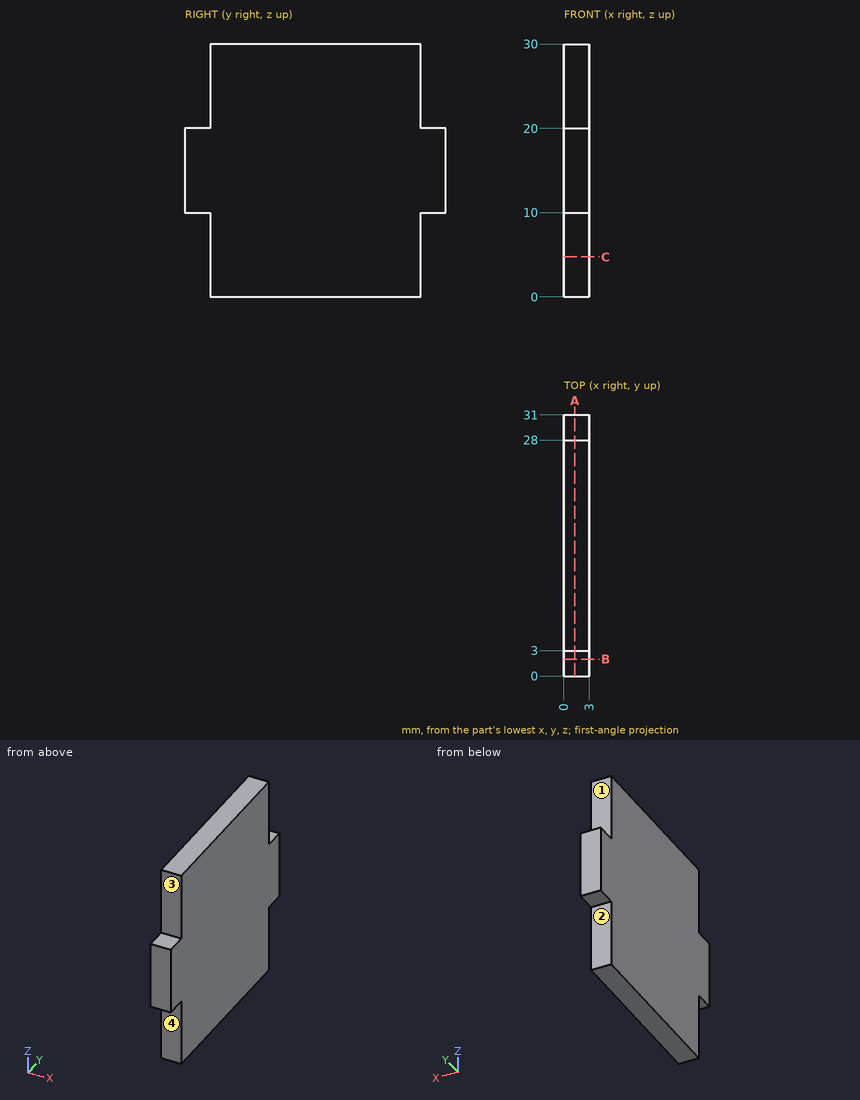
The figure shows three views and two pictorial views of one solid part (mm, origin at its lowest corner). Answer the questions. A direction names the side the tool comes from. Give positions to 0.01 mm unless a question says otherwise; leave off trailing zeros. Write each loop counter-clockwise with the first axis right and the second up, starting at its lowest first coordinate (ties: lowest second). Pieces come first, ordered by that corner, then holes. Notation, with made-up numbers: (-16.5, 63) - (-6.5, 63) arc R21 ccw to (-6.5, 78) - close; hole circle Ø11 at (33.25, 71.5). An arc over 180 degrees is marked (long way). Use one line per item in the form item = value. Start each with the question number.
1) A tool of negligible diameter and unlimited length cuts with its end or side. For the marked faces 1, 2, 3 and 4, from which of +Z, -Z, +X, -X, +Y, -Y can it reach the whole face along a straight path? Write none if from no direction.
2) Find section C-C on z = 4.75. Determine the outline of the cut face in (x, y), plus the area to 3 significant figures.
3) Find section B-B on y = 2. Determine the outline of the cut face in (x, z), plus the area to 3 significant figures.
4) Consider line 1 along Y through (x, z) = (0.5, 7.75); line 2 along Z through (x, y) = (0.65, 2). Determine where each line is inside the solid, lowest interval first. Write a range as from..to.
5) Find section A-A on x = 1.3. Determine the outline of the cut face in (y, z).
6) Flat-ended cylindrical pins translate along their axes: pin 1 Ø0.9 at (x, z) = (2, 3) entering from +Y; pin 2 Ø1.5 at (x, z) = (1, 22.5) entering from -Y. Find the tip coordinate at first contact, or state that the pin passes through.
Geometry results:
q1.face_1 = +Z, +X, -X, +Y
q1.face_2 = -Z, +X, -X, +Y
q1.face_3 = +Z, +X, -X, -Y
q1.face_4 = -Z, +X, -X, -Y
q2.outline = (0, 3) - (3, 3) - (3, 28) - (0, 28) - close
q2.area = 75.0 mm2
q3.outline = (0, 10) - (3, 10) - (3, 20) - (0, 20) - close
q3.area = 30.0 mm2
q4.line_1 = 3..28
q4.line_2 = 10..20
q5.outline = (0, 10) - (3, 10) - (3, 0) - (28, 0) - (28, 10) - (31, 10) - (31, 20) - (28, 20) - (28, 30) - (3, 30) - (3, 20) - (0, 20) - close
q6.pin_1 = 28
q6.pin_2 = 3
